Here's how the part is built. I have some questions about the finished solid (model axes, mm). A direction names the side the tool comes from. Give positions to 0.01 mm unless a question says otherwise; leave off trailing zeros. Order: outer loops, then holes, each group sorted by start corner. A loop starts at its lowest first (then second) coordinate and runs counter-clockwise, first axis right, second up. Notation, with made-up numbers: (30, 9.5) - (66, 9.5) arc R30 ccw to (66, 36.5) - close; hole circle Ø1 at (-3.75, 14). An arc over 180 degrees is marked (long way). One line per question, with ' | ' between items.
from build123d import *

# Parameters (mm, degrees)
SKETCH1_W           = 136.525
SKETCH1_H           = 787.4
BOSS_EXTRUDE1_DEPTH = 88.9
BOSS_EXTRUDE2_DEPTH = 25.4
SKETCH3_R           = 9.525
SKETCH3_R_2         = 15.875
CUT_EXTRUDE1_DEPTH  = 434.829216289
SKETCH5_W           = 44.45
SKETCH5_H           = 76.2
CUT_EXTRUDE2_DEPTH  = 19.05
SKETCH6_W           = 15.875
SKETCH6_H           = 69.85
SKETCH6_H_2         = 88.9
CUT_EXTRUDE3_DEPTH  = 50.8
SKETCH7_R           = 4.7625
CUT_EXTRUDE4_DEPTH  = 44.45
SKETCH7_3_R         = 6.35
CUT_EXTRUDE5_DEPTH  = 450.652194062
SKETCH8_R           = 14.2875
CUT_EXTRUDE6_DEPTH  = 12.7


with BuildPart() as part:
    # Sketch1 → Boss-Extrude1 (new body)
    with BuildSketch(Plane.XY):
        Rectangle(SKETCH1_W, SKETCH1_H)
    extrude(amount=BOSS_EXTRUDE1_DEPTH)

    # Sketch2 → Boss-Extrude2 (add)
    with BuildSketch(Plane(origin=(0, 393.7, 0), x_dir=(1, 0, 0), z_dir=(0, 1, 0))):
        Polygon((-42.8625, -60.325), (42.8625, -60.325), (42.8625, -15.875), (28.575, -15.875), (28.575, -41.275), (-1.5875, -41.275), (-1.5875, -15.875), (-42.8625, -15.875), align=None)
    extrude(amount=BOSS_EXTRUDE2_DEPTH)

    # Sketch3 → Cut-Extrude1 (cut, through all)
    with BuildSketch(Plane.XY.offset(88.9)):
        with Locations((0, 63.5)):
            Circle(SKETCH3_R)
        with Locations((0, -114.3)):
            Circle(SKETCH3_R)
        with Locations((0, 241.3)):
            Circle(SKETCH3_R)
        with Locations((7.9375, 323.85)):
            Circle(SKETCH3_R_2)
    extrude(amount=-CUT_EXTRUDE1_DEPTH, mode=Mode.SUBTRACT)

    # Sketch5 → Cut-Extrude2 (cut)
    with BuildSketch(Plane.ZY.offset(68.2625)):
        with Locations((38.1, -212.725)):
            Rectangle(SKETCH5_W, SKETCH5_H)
    extrude(amount=-CUT_EXTRUDE2_DEPTH, mode=Mode.SUBTRACT)

    # Sketch6 → Cut-Extrude3 (cut)
    with BuildSketch(Plane(origin=(0, 0, 0), x_dir=(-1, 0, 0), z_dir=(0, 0, -1))):
        with Locations((-46.0375, 339.725)):
            Rectangle(SKETCH6_W, SKETCH6_H)
        with Locations((-46.0375, -212.725)):
            Rectangle(SKETCH6_W, SKETCH6_H_2)
    extrude(amount=-CUT_EXTRUDE3_DEPTH, mode=Mode.SUBTRACT)

    # Sketch7 → Cut-Extrude4 (cut)
    with BuildSketch(Plane(origin=(68.2625, 0, 0), x_dir=(0, 0, -1), z_dir=(1, 0, 0))):
        with Locations(Location((-25.4, -236.5375, 0), (0, 0, 90))):
            Circle(SKETCH7_R)
        with Locations(Location((-25.4, -188.9125, 0), (0, 0, 90))):
            Circle(SKETCH7_R)
        with Locations(Location((-25.4, 315.9125, 0), (0, 0, 90))):
            Circle(SKETCH7_R)
        with Locations(Location((-25.4, 363.5375, 0), (0, 0, 90))):
            Circle(SKETCH7_R)
    extrude(amount=-CUT_EXTRUDE4_DEPTH, mode=Mode.SUBTRACT)

    # Sketch7_3 → Cut-Extrude5 (cut, through all)
    with BuildSketch(Plane(origin=(68.2625, 0, 0), x_dir=(0, 0, -1), z_dir=(1, 0, 0))):
        with Locations(Location((-25.4, -212.725, 0), (0, 0, 90))):
            Circle(SKETCH7_3_R)
    extrude(amount=-CUT_EXTRUDE5_DEPTH, mode=Mode.SUBTRACT)

    # Sketch8 → Cut-Extrude6 (cut)
    with BuildSketch(Plane(origin=(68.2625, 0, 0), x_dir=(0, 0, -1), z_dir=(1, 0, 0))):
        with Locations(Location((-25.4, -212.725, 0), (0, 0, 90))):
            Circle(SKETCH8_R)
    extrude(amount=-CUT_EXTRUDE6_DEPTH, mode=Mode.SUBTRACT)


solid = part.part
1) On a 3-axis mill with a long thin cutter (end or side, diameter ignored), from which of +Z, -Z, +X, -X, +Y, -Y can I reach the whole of each face in a straight line? I mean faces 5 (the face through (-59, -174.625, 38)), 6 (the face through (-22, 406, 15.875)), 7 (the face through (38.1, -203, 25)). Say none if no direction works.
Model answer:
face 5: -X | face 6: -Z, +X, -X, +Y | face 7: -Z
2) Thinking about a two-plate mould opening in Z: for faces 1 (the face through (55.562, -210, 19)), 2 (the face through (-4.945, -217.764, 21.536)), 3 (the face through (14, 406, 41.275)), 4 (the face through (-1, 406, 60.325)), which applies, +Z half, -Z half, draft (parallel to the pull), parting line (faces both ways), or undercut?
Model answer:
face 1: undercut | face 2: undercut | face 3: -Z half | face 4: +Z half
3) Please list where these lines run through material, in increasing order: L1, parallel to Y at x = 35, z = 25; L2, parallel to Y at x = 28, z = 25; L3, parallel to X at y = -244, z = 17 (1 decimal).
Model answer:
L1: y = -393.7 to -241.28, -231.79 to -219.06, -206.39 to -193.66, -184.17 to 311.17, 320.66 to 358.79, 368.28 to 419.1 | L2: y = -393.7 to -241.28, -231.79 to -219.06, -206.39 to -193.66, -184.17 to 311.17, 320.66 to 358.79, 368.28 to 393.7 | L3: x = -49.2 to 38.1, 54 to 68.3
4) I want a section at A-A (x = -24.5). List the corners of the cut face in (y, z) for me (3 decimals).
Model answer:
outline: (-393.7, 0) - (393.7, 0) - (393.7, 15.875) - (419.1, 15.875) - (419.1, 60.325) - (393.7, 60.325) - (393.7, 88.9) - (-393.7, 88.9) - close; hole circle Ø12.7 at (-212.725, 25.4)
5) I want a section at D-D (x = -59). List the corners of the cut face in (y, z) for me (3 decimals), plus the area to 3 significant figures.
Model answer:
outline: (-393.7, 0) - (393.7, 0) - (393.7, 88.9) - (-393.7, 88.9) - close; hole (-250.825, 15.875) - (-174.625, 15.875) - (-174.625, 60.325) - (-250.825, 60.325) - close | area: 66,600 mm2
6) I'm going to push flat-ended pins straight in: P1, Ø1, axis at x = 51, z = 69, coming from the +Y side; P2, Ø5, axis at y = -187.5, z = 26, coming from the +X side; P3, Ø20.5, axis at y = 412.5, z = 28.5, coming from the -X side. Where does each tip first touch, or does it pass through?
Model answer:
P1: stops at y = 393.7 | P2: stops at x = 23.81 | P3: stops at x = -42.86
7) I want a section at B-B (y = 63.5). List the corners of the cut face in (x, z) for me (1 decimal), plus the area to 3 significant figures.
Model answer:
outline: (-68.3, 0) - (-9.5, 0) - (-9.5, 88.9) - (-68.3, 88.9) - close; (9.5, 0) - (68.3, 0) - (68.3, 88.9) - (9.5, 88.9) - close | area: 10,400 mm2
8) I want a section at C-C (z = 68.5). State how many separate pieces and enclosed holes the cut face has, plus the area to 3 significant figures.
Model answer:
separate pieces: 1 | enclosed holes: 4 | area: 106,000 mm2
